Design review of the part built by this model. Coordinates are the model's own, in mm. A direction names the side the tool comes from. Give positions to 0.01 mm unless a question says otherwise; leave off trailing zeros. Write each loop counter-clockwise with the first axis right and the second up, starting at its lowest first coordinate (ties: lowest second). Pieces come first, ordered by that corner, then holes. Notation, with made-up numbers: M 85.25,42.25 L 105.25,42.25 A23 ccw 105.25,63.25 Z; hole C 84.25,62.5 d11. An arc over 180 degrees is marked long. Answer in a Markdown table with one row per item.
Autodesk Inventor part; units mm, degrees
ref_plane "YZ Plane" through (0, 0, 0) normal (1, 0, 0) x (0, 1, 0)
ref_plane "XZ Plane" through (0, 0, 0) normal (0, 1, 0) x (-1, 0, 0)
ref_plane "XY Plane" through (0, 0, 0) normal (0, 0, 1) x (1, 0, 0)
sketch "Sketch1" plane through (0, 0, 0) normal (0, 0, 1) x (1, 0, 0)
  line L0 (0, 0) -> (119, 0)
  line L1 (119, 0) -> (119, 80)
  line L2 (119, 80) -> (0, 80)
  line L3 (0, 80) -> (0, 0)
  dimension "d0" = 119
  dimension "d1" = 80
extrude "Extrusion1" add sketch "Sketch1" along normal blind 10
sketch "Sketch2" plane through (0, 0, 10) normal (0, 0, 1) x (1, 0, 0)
  circle A0 centre (109.5, 70) radius 2.5
  circle A1 centre (109.5, 10) radius 2.5
  line L0 (119, 80) -> (0, 80)
  line L1 (119, 0) -> (119, 80)
  point P0 (0, 0)
  dimension "d4" = 5
  dimension "d5" = 5
  dimension "d6" = 10
  dimension "d7" = 60
  dimension "d8" = 9.5
extrude "Extrusion2" cut sketch "Sketch2" against normal through all
sketch "Sketch3" plane through (0, 0, 0) normal (0, 0, -1) x (-1, 0, 0)
  line L0 (-119, 0) -> (-119, 80)
  line L1 (-119, 60) -> (-109, 60)
  line L2 (-109, 60) -> (-109, 20)
  line L3 (-109, 20) -> (-119, 20)
  line L4 (-119, 20) -> (-119, 60)
  line L5 (-119, 80) -> (0, 80)
  point P0 (0, 0)
  dimension "d11" = 10
  dimension "d12" = 40
  dimension "d13" = 20
extrude "Extrusion3" cut sketch "Sketch3" against normal blind 5
sketch "Sketch4" plane through (0, 0, 5) normal (0, 0, -1) x (-1, 0, 0)
  line L0 (-109, 60) -> (-119, 60)
  line L1 (-119, 60) -> (-119, 20)
  line L2 (-119, 20) -> (-109, 20)
  line L3 (-109, 20) -> (-109, 60)
  line L4 (-119, 80) -> (0, 80)
  line L5 (-119, 0) -> (-119, 80)
  circle A0 centre (-114, 40) radius 2.5
  point P0 (0, 0)
  point P1 (-119, 20)
  point P2 (-119, 40)
  point P3 (-114, 60)
  point P4 (-119, 40)
  dimension "d18" = 10
  dimension "d19" = 40
  dimension "d20" = 20
  dimension "d21" = 5
extrude "Extrusion4" cut sketch "Sketch4" against normal through all contours A0
sketch "Sketch5" plane through (0, 0, 10) normal (0, 0, 1) x (1, 0, 0)
  circle A0 centre (59.5, 70.5) radius 2.5
  line L0 (119, 80) -> (0, 80)
  point P0 (0, 0)
  point P1 (59.5, 80)
  dimension "d24" = 5
  dimension "d25" = 9.5
extrude "Extrusion5" cut sketch "Sketch5" against normal through all
properties part number "SP004" material "ABS Plastic"
1) Insertion check: P1, Ø1.5, axis at y = 46, z = 3.5, coming from the +X side; P2, Ø3, axis at x = 113, y = 31.5, coming from the -Z side. Each pin has a flat end and moves straight along its axis. Give the tip position at first contact, or say it passes through.
Geometry says:
| item | result |
|---|---|
| P1 | x = 109 |
| P2 | z = 5 |
2) To check wall thickness, follow probe 1 along Y at (x, z) = (109.5, 5.75); probe 2 along Y at (x, z) = (114, 7.2); probe 3 along Y at (x, z) = (59.5, 4.75). State the ranges of each line that lie inside material, in increasing order. Write a range as [from, to].
Geometry says:
| item | result |
|---|---|
| probe 1 | [0, 7.5], [12.5, 67.5], [72.5, 80] |
| probe 2 | [0, 37.5], [42.5, 80] |
| probe 3 | [0, 68], [73, 80] |
3) Add section C-C (z = 3.5). Write out the cut boundary in (x, y), and give its area (3 significant figures).
Geometry says:
| item | result |
|---|---|
| outline | M 0,0 L 119,0 L 119,20 L 109,20 L 109,60 L 119,60 L 119,80 L 0,80 Z; hole C 59.5,70.5 d5; hole C 109.5,10 d5; hole C 109.5,70 d5 |
| area | 9,060 mm^2 |
4) Add section D-D (y = 27.5). Write out the cut boundary in (x, z), and give its area (3 significant figures).
Geometry says:
| item | result |
|---|---|
| outline | M 0,0 L 109,0 L 109,5 L 119,5 L 119,10 L 0,10 Z |
| area | 1,140 mm^2 |
5) Add section B-B (y = 40). Write out the cut boundary in (x, z).
Geometry says:
| item | result |
|---|---|
| outline | M 0,0 L 109,0 L 109,5 L 111.5,5 L 111.5,10 L 0,10 Z; M 116.5,5 L 119,5 L 119,10 L 116.5,10 Z |
6) Add section A-A (x = 114). Write out the cut boundary in (y, z), and give its area (3 significant figures).
Geometry says:
| item | result |
|---|---|
| outline | M 0,0 L 20,0 L 20,5 L 37.5,5 L 37.5,10 L 0,10 Z; M 42.5,5 L 60,5 L 60,0 L 80,0 L 80,10 L 42.5,10 Z |
| area | 575 mm^2 |
7) For faces 5 (the face through (117, 40, 5)), 6 (the face through (111.885, 10.751, 5.07)), list the 3-axis set-ups (+Z, -Z, +X, -X, +Y, -Y) from which the entire face can be reached by the end or side of a thin tool; tool diameter is ignored.
Geometry says:
| item | result |
|---|---|
| face 5 | -Z, +X |
| face 6 | +Z, -Z |
8) The part is to be moulded in two halves that separate along X. For faces 1 (the face through (59, 41, 0)), 2 (the face through (0, 41, 5)), 3 (the face through (109, 40, 2)), 4 (the face through (61.81, 69.54, 5.07)), say which applies: released by +X, released by -X, zero draft, split by the parting line, or undercut.
Geometry says:
| item | result |
|---|---|
| face 1 | zero draft |
| face 2 | released by -X |
| face 3 | released by +X |
| face 4 | undercut |
